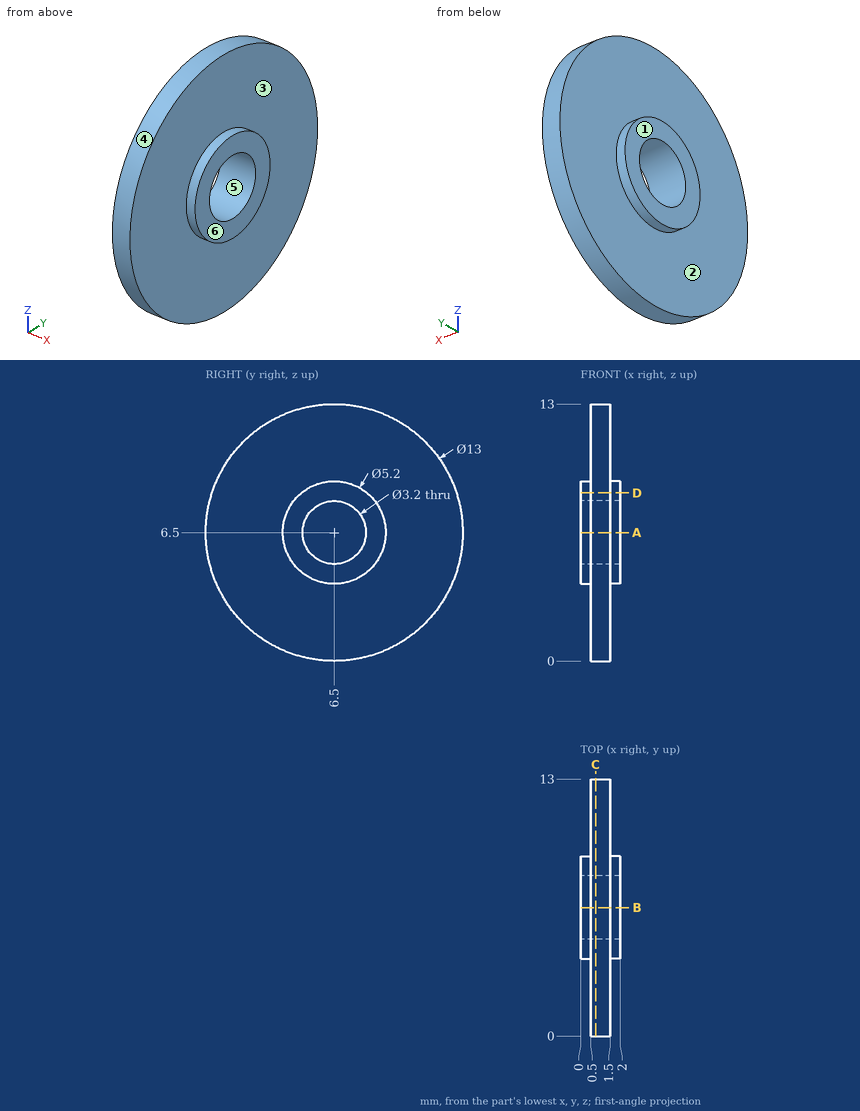
For this review, use the dimensioned drawing (mm, ordinates from the lowest corner) and the shaded views. A direction names the side the tool comes from. Coordinates: 2 decimals unless noted, no trailing zeros. Write each loop counter-clockwise with the first axis right and the second up, starting at its lowest first coordinate (ties: lowest second). Pieces come first, ordered by that corner, then holes. Notation, with made-up numbers: (17, 65.25) - (53, 65.25) arc R29 cw to (53, 103.25) - close; hole circle Ø5 at (4.5, 10). An arc over 180 degrees is marked (long way). Answer in a Markdown table with one row per item. Add a question column.
Q1. Consider section A-A on z = 6.5. Give the boundary of the cut face in (x, y), then the cut area to 3 significant figures.
Q2. Consider section C-C on x = 0.75. Give the boundary of the cut face in (y, z).
Q3. Consider section D-D on z = 8.5. Give the boundary of the cut face in (x, y).
Q4. Clearance check with a flat-ended pin moving along its axis: pin 1 (2 mm diameter, centred on y = 2.5, z = 11.5, fed in from -X). State where the tip first meets the part, or that it passes through.
Q5. For the marked faces 1, 2 and 3, list the 3-axis set-ups (+Z, -Z, +X, -X, +Y, -Y) from which the entire face can be reached by the end or side of a thin tool; tool diameter is ignored.
Q6. To check wall thickness, follow line 1 along Y through (x, z) = (0.9, 6.5); line 2 along Y through (x, z) = (0.35, 7.5). State the ranges of each line that lie inside material, in increasing order. Write a range as from..to.
Q7. Draft analysis for pull direction Y (two halves, no side actions). For the marked faces 4, 5 and 6, state which applies: +Y half, -Y half, draft (parallel to the pull), parting line (faces both ways), or undercut.
Answers below:
| question | item | result |
|---|---|---|
| 1 | outline | (0, 3.9) - (0.5, 3.9) - (0.5, 0) - (1.5, 0) - (1.5, 3.9) - (2, 3.9) - (2, 4.9) - (0, 4.9) - close; (0, 8.1) - (2, 8.1) - (2, 9.1) - (1.5, 9.1) - (1.5, 13) - (0.5, 13) - (0.5, 9.1) - (0, 9.1) - close |
| 1 | area | 11.8 mm² |
| 2 | outline | circle Ø13 at (6.5, 6.5); hole circle Ø3.2 at (6.5, 6.5) |
| 3 | outline | (0, 4.84) - (0.5, 4.84) - (0.5, 0.32) - (1.5, 0.32) - (1.5, 4.84) - (2, 4.84) - (2, 8.16) - (1.5, 8.16) - (1.5, 12.68) - (0.5, 12.68) - (0.5, 8.16) - (0, 8.16) - close |
| 4 | pin 1 | x = 0.5 |
| 5 | face 1 | +Z, -Z, -X, +Y, -Y |
| 5 | face 2 | -X |
| 5 | face 3 | +X |
| 6 | line 1 | 0..4.9, 8.1..13 |
| 6 | line 2 | 4.1..5.25, 7.75..8.9 |
| 7 | face 4 | parting line |
| 7 | face 5 | undercut |
| 7 | face 6 | draft |
